```python
from build123d import *

# Parameters (mm, degrees)
F0_W     = 2
F0_H     = 80
F1_ANGLE = 45
F2_DEPTH = 80
F4_DEPTH = 71.501
F5_SIZE  = 10


with BuildPart() as f1:
    # F0 (on Right) → F1 (revolve)
    with BuildSketch(Plane.YZ):
        with Locations((60, 0)):
            Rectangle(F0_W, F0_H)
    revolve(axis=Axis((0, 0, 0), (0, 0, -1)), revolution_arc=F1_ANGLE)

    # F2 (add): a face of the model
    f2_faces = [f1.faces().sort_by_distance(p)[0] for p in [
        (42.4264068712, 42.4264068712, 0),
    ]]
    extrude(f2_faces, amount=F2_DEPTH)

    # F3 (on face) → F4 (cut, through all)
    with BuildSketch(Plane(origin=(43.1335136524, 43.1335136524, 0), x_dir=(-0.7071067812, 0.7071067812, 0), z_dir=(0.7071067812, 0.7071067812, 0))):
        with BuildLine():
            ThreePointArc((20, -10), (30, 0), (20, 10))
            Line((20, 10), (-30, 10))
            ThreePointArc((-30, 10), (-40, 0), (-30, -10))
            Line((-30, -10), (20, -10))
        make_face()
    extrude(amount=-F4_DEPTH, mode=Mode.SUBTRACT)

    # F5
    f5_edges = [f1.edges().sort_by_distance(p)[0] for p in [
        (98.994949, -14.142136, 40),
        (98.994949, -14.142136, -40),
    ]]
    chamfer(f5_edges, length=F5_SIZE)


solid = f1.part
```
Geometry: final body of the model. Coordinates: model frame, mm. Coordinates: 2 decimals unless noted, no trailing zeros. Order: outer loops, then holes, each group sorted by start corner. A loop starts at its lowest first (then second) coordinate and runs counter-clockwise, first axis right, second up.
Item 1: Section query B-B (x = 49). Output: boundary loops of the cut face in (y, z).
Answer:
outline: (34.44, -40) - (37.27, -40) - (37.27, -10) - (34.44, -10) - close; (34.44, 10) - (37.27, 10) - (37.27, 40) - (34.44, 40) - close
Item 2: Section query A-A (y = 49.5). Output: boundary loops of the cut face in (x, z).
Answer:
outline: (32.11, -40) - (35.65, -40) - (35.65, -10) - (32.11, -10) - close; (32.11, 10) - (35.65, 10) - (35.65, 40) - (32.11, 40) - close
Item 3: Contact query for flat-ended pins moving along their axis: P1, Ø6, axis at y = 23, z = 7.5, coming from the +X side; P2, Ø8, axis at y = -4.5, z = -2.5, coming from the +X side; P3, Ø1.5, axis at x = 53.5, z = -28, coming from the -Y side. Output: stop coordinate, or through.
Answer:
P1: stops at x = 64.99
P2: stops at x = 94.77
P3: stops at y = 29.19
Item 4: Draft query along Z for faces 1 (the face through (95.4, -10.57, -35.07)), 2 (the face through (75.89, 7.55, -0.56)), 3 (the face through (95.499, -10.666, 34.93)), 4 (the face through (46, 38, -10)). Return one class per face: released by +Z, released by -Z, zero draft, split by the parting line, or undercut.
Answer:
face 1: released by -Z
face 2: zero draft
face 3: released by +Z
face 4: undercut
Item 5: Section query C-C (z = 25). Output: boundary loops of the cut face in (x, y).
Answer:
outline: (0, 59) arc R59 cw to (41.72, 41.72) - (98.29, -14.85) - (99.7, -13.44) - (43.13, 43.13) arc R61 ccw to (0, 61) - close
Item 6: Material intervals for line 1 along Y through (x, z) = (42, -24); line 2 along X through (y, z) = (45, 13); line 3 along X through (y, z) = (-3.5, 14), sorted ascending.
Answer:
line 1: y = 41.44 to 44.24
line 2: x = 38.16 to 41.18
line 3: x = 86.94 to 89.77
Item 7: Section query D-D (x = 76). Output: boundary loops of the cut face in (y, z).
Answer:
outline: (7.44, -40) - (10.27, -40) - (10.27, 40) - (7.44, 40) - close
